Here's how the part is built. I have some questions about the finished solid (model axes, mm). Coordinates: 2 decimals unless noted, no trailing zeros. Loops run counter-clockwise (first coordinate to the right, second up) from the corner with the lowest first, then second, coordinate; pieces in that order, holes last. Notation, with made-up numbers: (-37, -37) -> (7, -37) arc R22 cw to (7, -7) -> close; hole circle Ø7 at (21.5, 83.5). An arc over 180 degrees is marked (long way). Use CSV: the item, a comma, the result in double quotes. Start each with the question number.
from build123d import *

# Parameters (mm, degrees)
SKETCH_1_R          = 21
EXTRUDE_1_DEPTH     = 15
SKETCH_2_R          = 2
CUT_EXTRUDE_1_DEPTH = 34.271609519


with BuildPart() as part:
    # 草图1 → 凸台-拉伸1 (new body)
    with BuildSketch(Plane.XY):
        Circle(SKETCH_1_R)
    extrude(amount=EXTRUDE_1_DEPTH)

    # 草图2 → 切除-拉伸1 (cut, through all)
    with BuildSketch(Plane.XY.offset(15)):
        with Locations((0, 10)):
            Circle(SKETCH_2_R)
        with Locations((8.660254038, 5)):
            Circle(SKETCH_2_R)
        with Locations((8.660254038, -5)):
            Circle(SKETCH_2_R)
        with Locations((0, -10)):
            Circle(SKETCH_2_R)
        with Locations((-8.660254038, -5)):
            Circle(SKETCH_2_R)
        with Locations((-8.660254038, 5)):
            Circle(SKETCH_2_R)
    extrude(amount=-CUT_EXTRUDE_1_DEPTH, mode=Mode.SUBTRACT)


solid = part.part
1) I want a section at C-C, the plane z = 11.5. Please give me the cut outline in (x, y), plus the area to 3 significant figures.
2) I want a section at A-A, the plane x = 0. Please give me the cut outline in (y, z), plus the area to 3 significant figures.
3) I want a section at B-B, the plane y = -5. Please give me the cut outline in (x, z), plus the area to 3 significant figures.
4) Please list where these lines run through material, in increasing order: L1, parallel to Y at x = 7, z = 6.5; L2, parallel to Y at x = 9, z = 2.5; L3, parallel to X at y = 6, z = 5.25. Write a range as [from, to].
5) Thinking about a two-plate mould opening in Y: for faces 1 (the face through (0, 12, 8)), 2 (the face through (20.03, 6.31, 7.4)), 3 (the face through (0, 0, 0)), which applies, pulls with the +Y half, pulls with the -Y half, needs draft (parallel to the pull), parting line crosses it, or undercut?
6) I want a section at D-D, the plane y = 11.5. Please give me the cut outline in (x, z), plus the area to 3 significant figures.
7) For P1, Ø8, axis at x = -7, z = 5, coming from the -Y side; P2, Ø2.5, axis at x = -8.66, y = 5, coming from the +Z side; P3, Ø4, axis at x = -15, z = 4.5, coming from the +Y side; P4, Ø6.5, axis at x = 0, y = 10, coming from the +Z side, each with a flat end and sliding along its axis, tell me the tip position at first contact or that it passes through.
Return value:
1,outline,"circle Ø42 at (0, 0); hole circle Ø4 at (-8.66, -5); hole circle Ø4 at (-8.66, 5); hole circle Ø4 at (0, -10); hole circle Ø4 at (0, 10); hole circle Ø4 at (8.66, -5); hole circle Ø4 at (8.66, 5)"
1,area,"1,310 mm²"
2,outline,"(-21, 0) -> (-12, 0) -> (-12, 15) -> (-21, 15) -> close; (-8, 0) -> (8, 0) -> (8, 15) -> (-8, 15) -> close; (12, 0) -> (21, 0) -> (21, 15) -> (12, 15) -> close"
2,area,"510 mm²"
3,outline,"(-20.4, 0) -> (-10.66, 0) -> (-10.66, 15) -> (-20.4, 15) -> close; (-6.66, 0) -> (6.66, 0) -> (6.66, 15) -> (-6.66, 15) -> close; (10.66, 0) -> (20.4, 0) -> (20.4, 15) -> (10.66, 15) -> close"
3,area,"492 mm²"
4,L1,"y = [-19.8, -6.12], [-3.88, 3.88], [6.12, 19.8]"
4,L2,"y = [-18.97, -6.97], [-3.03, 3.03], [6.97, 18.97]"
4,L3,"x = [-20.12, -10.39], [-6.93, 6.93], [10.39, 20.12]"
5,face 1,"undercut"
5,face 2,"parting line crosses it"
5,face 3,"needs draft"
6,outline,"(-17.57, 0) -> (-1.32, 0) -> (-1.32, 15) -> (-17.57, 15) -> close; (1.32, 0) -> (17.57, 0) -> (17.57, 15) -> (1.32, 15) -> close"
6,area,"487 mm²"
7,P1,"stops at y = -20.78"
7,P2,"passes through"
7,P3,"stops at y = 16.49"
7,P4,"stops at z = 15"
